Geometry check sheet. Reference: drawing and pictorial views, mm from the part's lowest x, y, z. A direction names the side the tool comes from. Round coordinates to 2 decimals unless told otherwise and drop trailing zeros. Order: outer loops, then holes, each group sorted by start corner. A loop starts at its lowest first (then second) coordinate and runs counter-clockwise, first axis right, second up.
(1) Thickness scan on L1, parallel to Y at x = 7.5, z = 4.5; L2, parallel to Y at x = 7.5, z = 40; L3, parallel to Z at x = 5.5, y = 21.5. Record the ranges inside material, lowest first.
(2) Cross-section at A-A on z = 4.75. Enter the section's corners in (x, y) (1 decimal).
(3) Draft check along Z on the marked faces 1, 2, 3 and 4. Enter one of: pulls with the +Z half, pulls with the -Z half, needs draft (parallel to the pull), parting line crosses it, or undercut.
(4) Cross-section at D-D on y = 7.5. Enter the section's corners in (x, z).
(5) Gauge pin test, flat ends, axial feed: P1, Ø5, axis at x = 7.5, y = 7.5, coming from the +Z side; P2, Ø6, axis at x = 7, z = 36, coming from the -Y side; P3, Ø5, axis at x = 7, z = 21.5, coming from the -Y side; P4, Ø12, axis at y = 30.5, z = 30, coming from the -X side. Record the tip position at first contact, or that the pin passes through.
(6) Set-up check for the marked faces 5 and 6: record each of +Z, -Z, +X, -X, +Y, -Y from which the full face is reachable in a straight line by a thin tool's end or side.
(7) Cross-section at C-C on y = 20.5. Enter the section's corners in (x, z), and give its area (3 significant figures).
(8) Cross-section at B-B on x = 7.5. Enter the section's corners in (y, z), and give its area (3 significant figures).
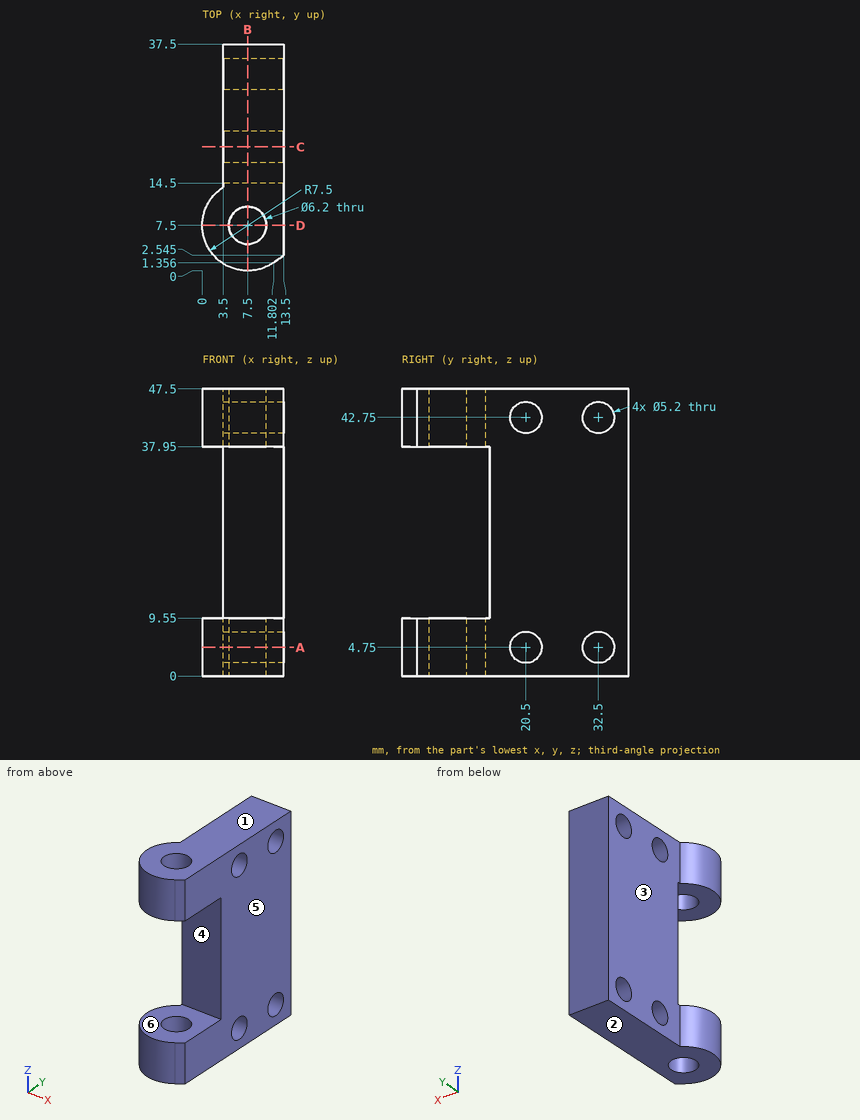
Found:
1. L1: y = 0 to 4.4, 10.6 to 17.91, 23.09 to 29.91, 35.09 to 37.5
1. L2: y = 0 to 4.4, 10.6 to 37.5
1. L3: z = 0 to 2.35, 7.15 to 40.35, 45.15 to 47.5
2. outline: (3.5, 13.8) arc R7.5 ccw (long way) to (11.8, 1.4) - (13.5, 2.5) - (13.5, 17.9) - (3.5, 17.9) - close; (3.5, 23.1) - (13.5, 23.1) - (13.5, 29.9) - (3.5, 29.9) - close; (3.5, 35.1) - (13.5, 35.1) - (13.5, 37.5) - (3.5, 37.5) - close; hole circle Ø6.2 at (7.5, 7.5)
3. face 1: pulls with the +Z half
3. face 2: pulls with the -Z half
3. face 3: needs draft
3. face 4: undercut
4. outline: (0, 0) - (4.4, 0) - (4.4, 9.55) - (0, 9.55) - close; (0, 37.95) - (4.4, 37.95) - (4.4, 47.5) - (0, 47.5) - close; (10.6, 0) - (13.5, 0) - (13.5, 9.55) - (10.6, 9.55) - close; (10.6, 37.95) - (13.5, 37.95) - (13.5, 47.5) - (10.6, 47.5) - close
5. P1: passes through
5. P2: stops at y = 0
5. P3: stops at y = 14.5
5. P4: stops at x = 3.5
6. face 5: +Z, -Z, +X, +Y, -Y
6. face 6: +X, -X, -Y
7. outline: (3.5, 0) - (13.5, 0) - (13.5, 2.15) - (3.5, 2.15) - close; (3.5, 7.35) - (13.5, 7.35) - (13.5, 40.15) - (3.5, 40.15) - close; (3.5, 45.35) - (13.5, 45.35) - (13.5, 47.5) - (3.5, 47.5) - close
7. area: 371 mm2
8. outline: (0, 0) - (4.4, 0) - (4.4, 9.55) - (0, 9.55) - close; (0, 37.95) - (4.4, 37.95) - (4.4, 47.5) - (0, 47.5) - close; (10.6, 0) - (37.5, 0) - (37.5, 47.5) - (10.6, 47.5) - (10.6, 37.95) - (14.5, 37.95) - (14.5, 9.55) - (10.6, 9.55) - close; hole circle Ø5.2 at (20.5, 4.75); hole circle Ø5.2 at (20.5, 42.75); hole circle Ø5.2 at (32.5, 4.75); hole circle Ø5.2 at (32.5, 42.75)
8. area: 1,170 mm2
